Source: three-view drawing plus pictorial views. Frame: mm from the lowest corner of the part. Coordinates: 2 decimals unless noted, no trailing zeros. Write each loop counter-clockwise with the first axis right and the second up, starting at its lowest first coordinate (ties: lowest second). Pieces come first, ordered by that corner, then holes. Notation, with made-up numbers: (-3.75, 87.5) - (8.25, 87.5) arc R11 ccw to (8.25, 96.5) - close; hole circle Ø5 at (-1, 31.25). An arc over 180 degrees is marked (long way). Put each result on its own line as item: value.
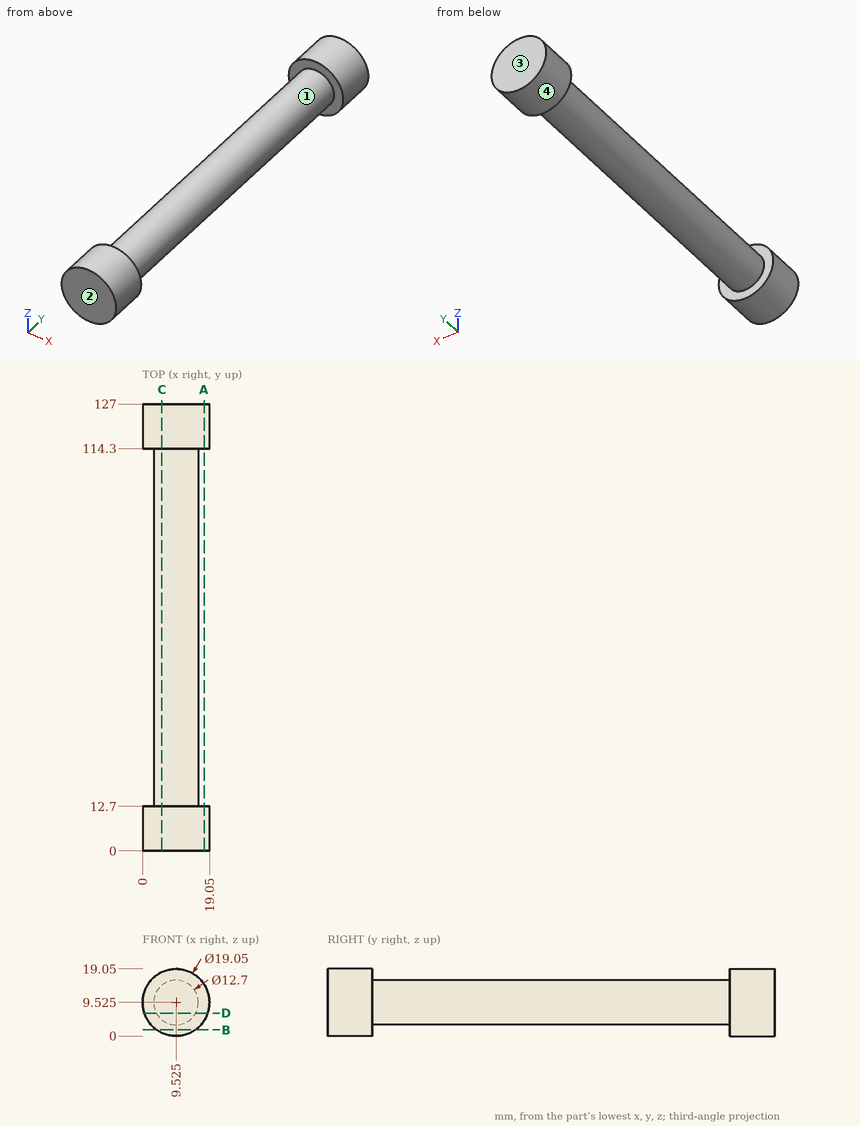
1. Ray query, probe 1 along Y at (x, z) = (15.25, 17); probe 2 along Z at (x, y) = (9, 13.5); probe 3 along Z at (x, y) = (9.75, 120). Return the intervals inside material, ascending. Write a range as from..to.
Answer below:
probe 1: y = 0..12.7, 114.3..127
probe 2: z = 3.2..15.85
probe 3: z = 0..19.05
2. Pin query (flat end, axial travel): pin 1 Ø3 at (x, y) = (11, 30.5) entering from +Z (3 decimals); pin 2 Ø1.5 at (y, z) = (18.5, 5) entering from -X; pin 3 Ø4 at (y, z) = (75.5, 7) entering from -X. Return the tip coordinate at first contact, or that it passes through.
Answer below:
pin 1: stops at z = 15.875
pin 2: stops at x = 4.42
pin 3: stops at x = 3.2
3. Section query C-C (x = 5.5). Return loops of the section in (y, z).
Answer below:
outline: (0, 0.89) - (12.7, 0.89) - (12.7, 4.61) - (114.3, 4.61) - (114.3, 0.89) - (127, 0.89) - (127, 18.16) - (114.3, 18.16) - (114.3, 14.44) - (12.7, 14.44) - (12.7, 18.16) - (0, 18.16) - close
4. Mould query, pull axis Y, two halves, no side actions, for the marked faces 1, 2, 3 and 4. Classes: +Y half, -Y half, draft (parallel to the pull), parting line (faces both ways), or undercut.
Answer below:
face 1: undercut
face 2: -Y half
face 3: +Y half
face 4: draft
5. Section query D-D (z = 6.5). Return loops of the section in (x, y), then the cut area to 3 significant figures.
Answer below:
outline: (0.49, 0) - (18.56, 0) - (18.56, 12.7) - (15.11, 12.7) - (15.11, 114.3) - (18.56, 114.3) - (18.56, 127) - (0.49, 127) - (0.49, 114.3) - (3.94, 114.3) - (3.94, 12.7) - (0.49, 12.7) - close
area: 1,590 mm²
6. Section query A-A (x = 17.5). Return loops of the section in (y, z).
Answer below:
outline: (0, 4.32) - (12.7, 4.32) - (12.7, 14.73) - (0, 14.73) - close; (114.3, 4.32) - (127, 4.32) - (127, 14.73) - (114.3, 14.73) - close
7. Section query B-B (z = 1.75). Return loops of the section in (x, y).
Answer below:
outline: (4.02, 0) - (15.03, 0) - (15.03, 12.7) - (4.02, 12.7) - close; (4.02, 114.3) - (15.03, 114.3) - (15.03, 127) - (4.02, 127) - close
